```python
from build123d import *

# Parameters (mm, degrees)
F0_W     = 150
F0_H     = 15
F1_DEPTH = 1
F2_W     = 2
F2_H     = 15
F3_DEPTH = 25
F4_R     = 3
F5_DEPTH = 2.001
F6_R     = 3
F7_DEPTH = 2.001


with BuildPart() as f1:
    # F0 (on Front) → F1 (new body, symmetric)
    with BuildSketch(Plane.XZ):
        with Locations((67.5, 0)):
            Rectangle(F0_W, F0_H)
        with BuildLine():
            ThreePointArc((0, -3), (-3, 0), (0, 3))
            Line((0, 3), (80, 3))
            ThreePointArc((80, 3), (83, 0), (80, -3))
            Line((80, -3), (0, -3))
        make_face(mode=Mode.SUBTRACT)
        with BuildLine():
            ThreePointArc((135, 3), (138, 0), (135, -3))
            ThreePointArc((135, -3), (132, 0), (135, 3))
        make_face(mode=Mode.SUBTRACT)
    extrude(amount=F1_DEPTH, both=True)

    # F2 (on face) → F3 (join)
    with BuildSketch(Plane.YZ.offset(142.5)):
        Rectangle(F2_W, F2_H)
    extrude(amount=F3_DEPTH)

    # F4 (on face) → F5 (cut, through all)
    with BuildSketch(Plane.XZ.offset(1)):
        with Locations((160, 0)):
            Circle(F4_R)
    extrude(amount=-F5_DEPTH, mode=Mode.SUBTRACT)

    # F6 (on face) → F7 (cut, through all)
    with BuildSketch(Plane.XZ.offset(1)):
        with Locations((115, 0)):
            Circle(F6_R)
    extrude(amount=-F7_DEPTH, mode=Mode.SUBTRACT)


solid = f1.part
```
CAD build for the part. Positions are in the model's coordinates, mm. A direction names the side the tool comes from. Round coordinates to 2 decimals unless told otherwise and drop trailing zeros. Write each loop counter-clockwise with the first axis right and the second up, starting at its lowest first coordinate (ties: lowest second). Pieces come first, ordered by that corner, then holes. Notation, with made-up numbers: M -35,72 L 21,72 A16 cw 21,100 Z; hole C 6,-8 d3. An arc over 180 degrees is marked long. One line per question, with ' | ' between items.
1. Probe L1, parallel to Z at x = 135, y = 0.55; L2, parallel to X at y = 0.7, z = -1.25. List the from-to ranges inside material, lowest first. Write a range as from..to.
Working result:
L1: -7.5..-3, 3..7.5 | L2: -7.5..-2.73, 82.73..112.27, 117.73..132.27, 137.73..157.27, 162.73..167.5
2. Which spindle directions (+Z, -Z, +X, -X, +Y, -Y) get a long thin tool onto all of the face, cutting with end or side? Do faces 3 (the flat face through (78.8, -1, -3.4)), 4 (the cylindrical face through (-3, 0, 0)). Say none if no direction does.
Working result:
face 3: +Z, -Z, +X, -X, -Y | face 4: +Y, -Y
3. Cut at A-A on x = 135. Write the cut outline in (y, z), and give its area (3 significant figures).
Working result:
outline: M -1,-7.5 L 1,-7.5 L 1,-3 L -1,-3 Z; M -1,3 L 1,3 L 1,7.5 L -1,7.5 Z | area: 18.0 mm2
4. Pin check, flat tip, straight feed: pin 1 Ø5.5 at (x, z) = (115, 0) entering from -Y. Stop position of the tip, or through.
Working result:
pin 1: through
5. Mould opens along X. For faces 1 (the flat face through (78.8, 1, -3.4)), 2 (the cylindrical face through (83, 0, 0)) say: pulls with the +X half, pulls with the -X half, needs draft (parallel to the pull), parting line crosses it, or undercut.
Working result:
face 1: needs draft | face 2: undercut
6. Cut at B-B on y = 0.55. Write the cut outline in (x, z).
Working result:
outline: M -7.5,-7.5 L 167.5,-7.5 L 167.5,7.5 L -7.5,7.5 Z; hole M 0,-3 L 80,-3 A3 ccw 80,3 L 0,3 A3 ccw Z; hole C 115,0 d6; hole C 135,0 d6; hole C 160,0 d6
